Check sheet for the modelled part. Datum: model origin and axes. Units: mm. Coordinates: 2 decimals unless noted, no trailing zeros. Write each loop counter-clockwise with the first axis right and the second up, starting at its lowest first coordinate (ties: lowest second). Pieces come first, ordered by that corner, then holes. Notation, with made-up numbers: (-17, 3.5) - (13, 3.5) arc R13 ccw to (13, 22.5) - close; hole circle Ø5 at (7, 10). An arc over 180 degrees is marked (long way). Use one line per item in the form item = value. Start each with the question number.
1. Scan lines: line 1 along Z through (x, y) = (-54, -3.4); line 2 along Z through (x, y) = (-53, -1.9). Record each from-to range of solid material in increasing order.
2. Go/stop test with flat-tipped pins: pin 1 Ø1 at (x, y) = (-67, -0.5) entering from +Z; pin 2 Ø1 at (x, y) = (-38, -1) entering from +Z. Record where each tip stops, or that it passes through.
3. Cross-section at B-B on y = -2.15. Record the boundary of the cut face in (x, z).
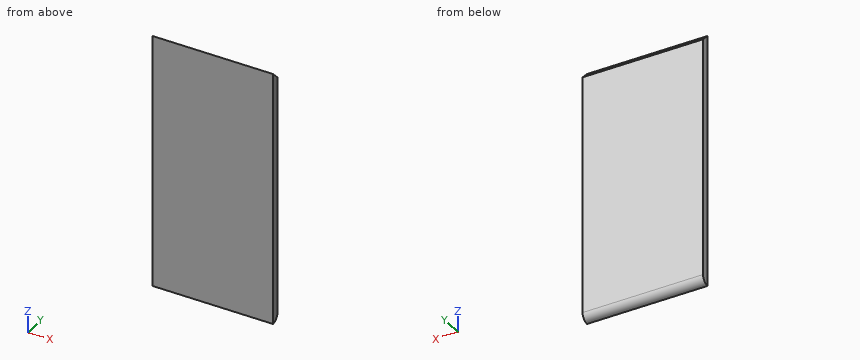
```python
from build123d import *

# Parameters (mm, degrees)
F0_W     = 80
F0_H     = 169.70563
F1_DEPTH = 5
F2_SIZE  = 4.99999
F3_R     = 4.99999


# Not quite as in the source:
# - a fillet or chamfer is up to 0.001 mm smaller than in the source, because OpenCascade refuses the exact size


with BuildPart() as f1:
    # F0 (on Front) → F1 (new body)
    with BuildSketch(Plane.XZ):
        with Locations((-37.0779657288, 20.5572328247)):
            Rectangle(F0_W, F0_H)
    extrude(amount=F1_DEPTH)

    # F2 (size 5 in the source; OpenCascade refuses exactly that, so slightly less here)
    f2_edges = [f1.edges().sort_by_distance(p)[0] for p in [
        (-37.077966, 0, 105.410048),
    ]]
    chamfer(f2_edges, length=F2_SIZE)

    # F3 (radius 5 in the source; OpenCascade refuses exactly that, so slightly less here)
    f3_edges = [f1.edges().sort_by_distance(p)[0] for p in [
        (-37.077966, 0, -64.295582),
    ]]
    fillet(f3_edges, radius=F3_R)


solid = f1.part
```
Final values:
q1.line_1 = -64.03 to 103.81
q1.line_2 = -63.22 to 102.31
q2.pin_1 = 101.41
q2.pin_2 = 101.91
q3.outline = (-77.08, -63.4) - (2.92, -63.4) - (2.92, 102.56) - (-77.08, 102.56) - close
